Part model, mm, in its own coordinate system. A direction names the side the tool comes from. Coordinates: 2 decimals unless noted, no trailing zeros. Write each loop counter-clockwise with the first axis right and the second up, starting at its lowest first coordinate (ties: lowest second). Pieces come first, ordered by that corner, then holes. Notation, with made-up numbers: (3, 72.5) - (10, 72.5) arc R17 ccw to (10, 89.5) - close; hole circle Ø7 at (81.5, 29.5). An arc over 180 degrees is marked (long way). Use one line per item in the form item = value. Start each with the question number.
from build123d import *

# Parameters (mm, degrees)
F0_W     = 82.55
F0_H     = 82.55
F0_W_2   = 57.15
F0_H_2   = 57.15
F1_DEPTH = 6.35
F2_W     = 82.55
F2_H     = 82.55
F2_W_2   = 76.2
F2_H_2   = 76.2
F3_DEPTH = 19.05
F4_W     = 82.55
F4_H     = 82.55
F4_W_2   = 69.85
F4_H_2   = 69.85
F5_DEPTH = 3.175
F6_R     = 5.08
F7_R     = 5.08


with BuildPart() as f1:
    # F0 (on Front) → F1 (new body)
    with BuildSketch(Plane.XZ):
        Rectangle(F0_W, F0_H)
        Rectangle(F0_W_2, F0_H_2, mode=Mode.SUBTRACT)
    extrude(amount=F1_DEPTH)

    # F2 (on face) → F3 (join)
    with BuildSketch(Plane(origin=(0, 0, 0), x_dir=(-1, 0, 0), z_dir=(0, 1, 0))):
        Rectangle(F2_W, F2_H)
        Rectangle(F2_W_2, F2_H_2, mode=Mode.SUBTRACT)
    extrude(amount=F3_DEPTH)

    # F4 (on face) → F5 (join)
    with BuildSketch(Plane(origin=(0, 19.05, 0), x_dir=(-1, 0, 0), z_dir=(0, 1, 0))):
        Rectangle(F4_W, F4_H)
        Rectangle(F4_W_2, F4_H_2, mode=Mode.SUBTRACT)
    extrude(amount=F5_DEPTH)

    # F6
    f6_edges = [f1.edges().sort_by_distance(p)[0] for p in [
        (41.275, 7.9375, -41.275),
        (41.275, 7.9375, 41.275),
        (-41.275, 7.9375, 41.275),
        (-41.275, 7.9375, -41.275),
    ]]
    fillet(f6_edges, radius=F6_R)

    # F7
    f7_edges = [f1.edges().sort_by_distance(p)[0] for p in [
        (-28.575, -3.175, -28.575),
        (28.575, -3.175, -28.575),
        (28.575, -3.175, 28.575),
        (-28.575, -3.175, 28.575),
    ]]
    fillet(f7_edges, radius=F7_R)


solid = f1.part
Q1. Slice it at B-B (x = -20.5). List the corners of the cut face in (y, z) (3 decimals), plus the area to 3 significant figures.
Q2. Slice it at C-C (y = -4.5). List the corners of the cut face in (x, z) (3 decimals).
Q3. Which spindle directions (+Z, -Z, +X, -X, +Y, -Y) get a long thin tool onto all of the face, cutting with end or side? Do faces 1 (the cylindrical face through (27.126, -3.219, 27.047)), 2 (the flat face through (0, 21, -34.925)), 3 (the flat face through (-37, -6.35, 1)). Say none if no direction does.
Q4. Slice it at A-A (z = -13). List the corners of the cut face in (x, y) (3 decimals), plus the area to 3 significant figures.
Q5. Slice it at D-D (x = 32). List the corners of the cut face in (y, z) (3 decimals).
Q6. Mould opens along Y. For faces 4 (the flat face through (37, 22.225, 1)), 5 (the flat face through (0, -3, 28.575)), 6 (the flat face through (3, 19.05, -37)) say: released by +Y, released by -Y, zero draft, split by the parting line, or undercut.
Q7. Drill centre lines: probe 1 along X at (y, z) = (9.75, 30.5) (3 decimals); probe 2 along Z at (x, y) = (-11, -2.5) (3 decimals). Where is each one in solid material? Low to high.
Solution:
q1.outline = (-6.35, -41.275) - (22.225, -41.275) - (22.225, -34.925) - (19.05, -34.925) - (19.05, -38.1) - (0, -38.1) - (0, -28.575) - (-6.35, -28.575) - close; (-6.35, 28.575) - (0, 28.575) - (0, 38.1) - (19.05, 38.1) - (19.05, 34.925) - (22.225, 34.925) - (22.225, 41.275) - (-6.35, 41.275) - close
q1.area = 323 mm2
q2.outline = (-41.275, -36.195) arc R5.08 ccw to (-36.195, -41.275) - (36.195, -41.275) arc R5.08 ccw to (41.275, -36.195) - (41.275, 36.195) arc R5.08 ccw to (36.195, 41.275) - (-36.195, 41.275) arc R5.08 ccw to (-41.275, 36.195) - close; hole (-28.575, -23.495) arc R5.08 ccw to (-23.495, -28.575) - (23.495, -28.575) arc R5.08 ccw to (28.575, -23.495) - (28.575, 23.495) arc R5.08 ccw to (23.495, 28.575) - (-23.495, 28.575) arc R5.08 ccw to (-28.575, 23.495) - close
q3.face_1 = +Y, -Y
q3.face_2 = +Y
q3.face_3 = +Z, -Z, +X, -X, -Y
q4.outline = (-41.275, -6.35) - (-28.575, -6.35) - (-28.575, 0) - (-38.1, 0) - (-38.1, 19.05) - (-34.925, 19.05) - (-34.925, 22.225) - (-41.275, 22.225) - close; (28.575, -6.35) - (41.275, -6.35) - (41.275, 22.225) - (34.925, 22.225) - (34.925, 19.05) - (38.1, 19.05) - (38.1, 0) - (28.575, 0) - close
q4.area = 323 mm2
q5.outline = (-6.35, -41.275) - (22.225, -41.275) - (22.225, -34.925) - (19.05, -34.925) - (19.05, -38.1) - (0, -38.1) - (0, 38.1) - (19.05, 38.1) - (19.05, 34.925) - (22.225, 34.925) - (22.225, 41.275) - (-6.35, 41.275) - close
q6.face_4 = released by +Y
q6.face_5 = zero draft
q6.face_6 = undercut
q7.probe_1 = -41.275 to -38.1, 38.1 to 41.275
q7.probe_2 = -41.275 to -28.575, 28.575 to 41.275
